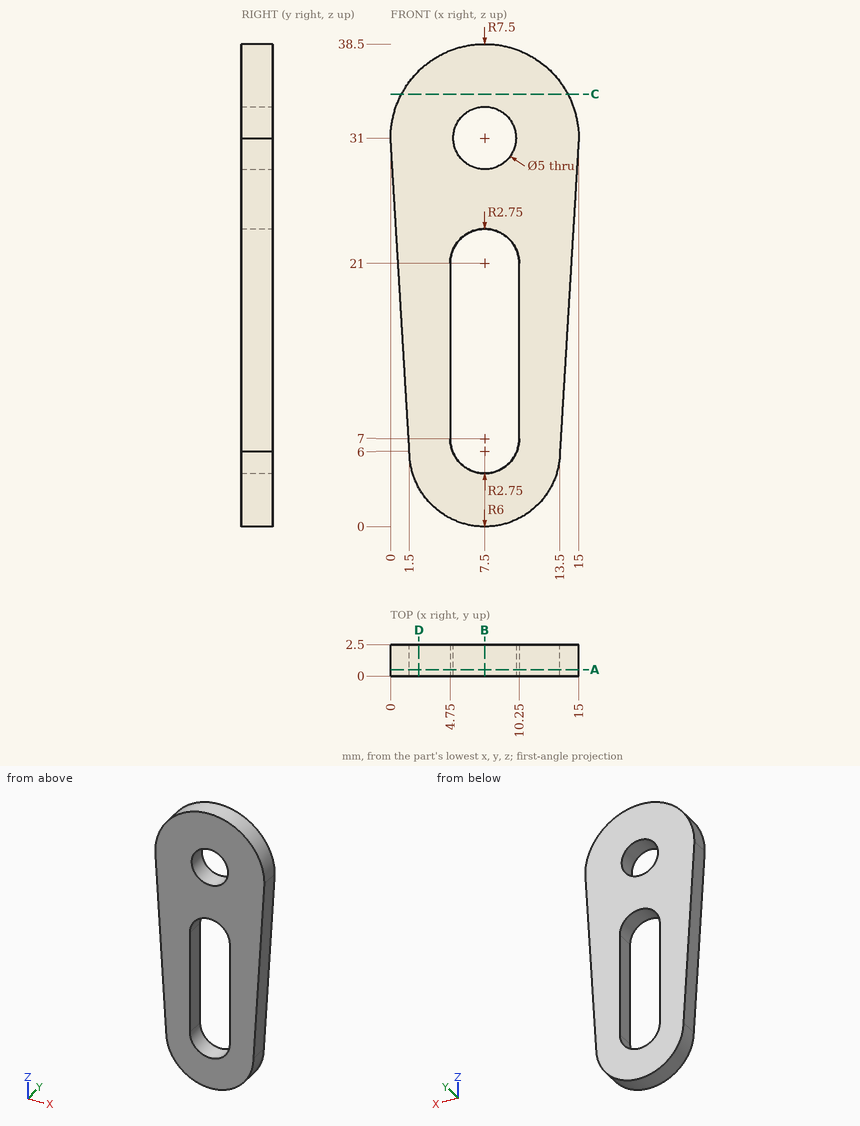
Geometry check sheet. Reference: drawing and pictorial views, mm from the part's lowest x, y, z. Round coordinates to 2 decimals unless told otherwise and drop trailing zeros. Order: outer loops, then holes, each group sorted by start corner. A loop starts at its lowest first (then second) coordinate and runs counter-clockwise, first axis right, second up. Notation, with made-up numbers: (-17.75, 71.5) - (-5.75, 71.5) arc R32 cw to (-5.75, 103.5) - close; hole circle Ø8 at (-12, -29). An arc over 180 degrees is marked (long way). Use a Markdown table: item, result. Add a question column.
1) Section check A-A (y = 0.5). Record the cut outline in (x, z), then the cut area to 3 significant figures.
2) Section check C-C (z = 34.5). Record the cut outline in (x, y), then the cut area to 3 significant figures.
3) Thickness scan on line 1 along Z through (x, y) = (7.5, 1.15); line 2 along X through (y, z) = (0.7, 31); line 3 along Z through (x, y) = (7, 1.8). Record the ranges inside material, lowest first.
4) Section check B-B (x = 7.5). Record the cut outline in (y, z).
5) Section check D-D (x = 2.25). Record the cut outline in (y, z), then the cut area to 3 significant figures.
6) Gauge pin test, flat ends, axial feed: P1, Ø1.5, axis at x = 3.5, z = 20.5, coming from the -Y side; P2, Ø0.8, axis at y = 1.5, z = 11.5, coming from the -X side. Record the tip position at first contact, or that the pin passes through.
Established:
| question | item | result |
|---|---|---|
| 1 | outline | (0, 31) - (1.5, 6) arc R6 ccw to (13.5, 6) - (15, 31) arc R7.5 ccw to start; hole (4.75, 7) arc R2.75 ccw to (10.25, 7) - (10.25, 21) arc R2.75 ccw to (4.75, 21) - close; hole circle Ø5 at (7.5, 31) |
| 1 | area | 362 mm2 |
| 2 | outline | (0.87, 0) - (14.13, 0) - (14.13, 2.5) - (0.87, 2.5) - close |
| 2 | area | 33.2 mm2 |
| 3 | line 1 | 0 to 4.25, 23.75 to 28.5, 33.5 to 38.5 |
| 3 | line 2 | 0 to 5, 10 to 15 |
| 3 | line 3 | 0.02 to 4.3, 23.7 to 28.55, 33.45 to 38.48 |
| 4 | outline | (0, 0) - (2.5, 0) - (2.5, 4.25) - (0, 4.25) - close; (0, 23.75) - (2.5, 23.75) - (2.5, 28.5) - (0, 28.5) - close; (0, 33.5) - (2.5, 33.5) - (2.5, 38.5) - (0, 38.5) - close |
| 5 | outline | (0, 3.1) - (2.5, 3.1) - (2.5, 36.36) - (0, 36.36) - close |
| 5 | area | 83.2 mm2 |
| 6 | P1 | y = 0 |
| 6 | P2 | x = 1.15 |
